from build123d import *

# Parameters (mm, degrees)
SKETCH_1_R          = 102
EXTRUDE_1_DEPTH     = 12
SKETCH_2_R          = 69
EXTRUDE_2_DEPTH     = 3
CUT_EXTRUDE_START   = -4
SKETCH_3_R          = 82
SKETCH_3_R_2        = 69
CUT_EXTRUDE_2_DEPTH = 4
SKETCH_4_R          = 63.75
EXTRUDE_3_DEPTH     = 1
CHAMFER_1_SIZE      = 0.5
SKETCH_5_R          = 5
CUT_EXTRUDE_3_DEPTH = 41
SKETCH_6_R          = 55
CUT_EXTRUDE_4_DEPTH = 51
SKETCH_7_R          = 4
CUT_EXTRUDE_5_DEPTH = 8


with BuildPart() as part:
    # 草图1 → 拉伸1 (new body)
    with BuildSketch(Plane.XY):
        Circle(SKETCH_1_R)
    extrude(amount=EXTRUDE_1_DEPTH)

    # 草图2 → 拉伸2 (add)
    with BuildSketch(Plane.XY.offset(12)):
        Circle(SKETCH_2_R)
    extrude(amount=EXTRUDE_2_DEPTH)

    # 草图3 → 切除-拉伸2 (cut)
    with BuildSketch(Plane.XY.offset(12).offset(CUT_EXTRUDE_START)):
        Circle(SKETCH_3_R)
        Circle(SKETCH_3_R_2, mode=Mode.SUBTRACT)
    extrude(amount=CUT_EXTRUDE_2_DEPTH, mode=Mode.SUBTRACT)

    # 草图4 → 拉伸3 (add)
    with BuildSketch(Plane.XY.offset(15)):
        Circle(SKETCH_4_R)
    extrude(amount=EXTRUDE_3_DEPTH)

    # 倒角1
    chamfer_1_edges = [part.edges().sort_by_distance(p)[0] for p in [
        (-82, 0, 12),
        (-102, 0, 0),
        (-102, 0, 12),
        (-69, 0, 15),
    ]]
    chamfer(chamfer_1_edges, length=CHAMFER_1_SIZE)

    # 草图5 → 切除-拉伸3 (cut)
    with BuildSketch(Plane(origin=(0, 0, 0), x_dir=(-1, 0, 0), z_dir=(0, 0, -1))):
        with Locations((0, 90)):
            Circle(SKETCH_5_R)
        with Locations((77.942286341, 45)):
            Circle(SKETCH_5_R)
        with Locations((77.942286341, -45)):
            Circle(SKETCH_5_R)
        with Locations((0, -90)):
            Circle(SKETCH_5_R)
        with Locations((-77.942286341, -45)):
            Circle(SKETCH_5_R)
        with Locations((-77.942286341, 45)):
            Circle(SKETCH_5_R)
    extrude(amount=-CUT_EXTRUDE_3_DEPTH, mode=Mode.SUBTRACT)

    # 草图6 → 切除-拉伸4 (cut)
    with BuildSketch(Plane(origin=(0, 0, 0), x_dir=(-1, 0, 0), z_dir=(0, 0, -1))):
        Circle(SKETCH_6_R)
    extrude(amount=-CUT_EXTRUDE_4_DEPTH, mode=Mode.SUBTRACT)

    # 草图7 → 切除-拉伸5 (cut)
    with BuildSketch(Plane(origin=(0, 0, 0), x_dir=(-1, 0, 0), z_dir=(0, 0, -1))):
        with Locations((51.265241636, 51.265241636)):
            Circle(SKETCH_7_R)
        with Locations((51.265241636, -51.265241636)):
            Circle(SKETCH_7_R)
        with Locations((-51.265241636, -51.265241636)):
            Circle(SKETCH_7_R)
        with Locations((-51.265241636, 51.265241636)):
            Circle(SKETCH_7_R)
    extrude(amount=-CUT_EXTRUDE_5_DEPTH, mode=Mode.SUBTRACT)


solid = part.part
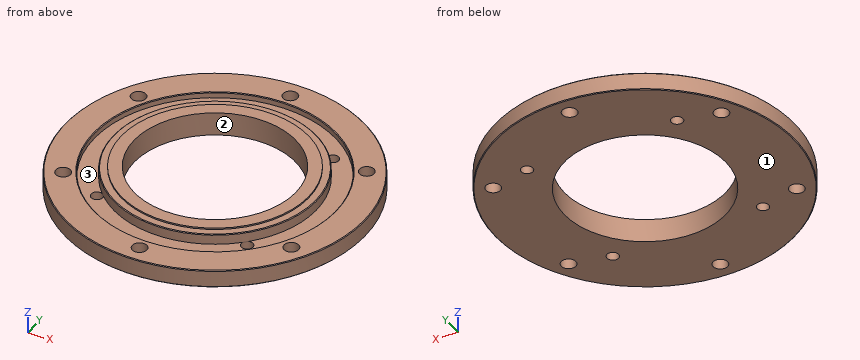
For this review, take the finished solid that the model builds, in its own axes (mm). Face numbers are marked on the shaded views. Round coordinates to 2 decimals unless told otherwise and drop trailing zeros. Loops run counter-clockwise (first coordinate to the right, second up) from the corner with the lowest first, then second, coordinate; pieces in that order, holes last. Notation, with made-up numbers: (-4.5, 66) - (8.5, 66) arc R25 cw to (8.5, 84) - close; hole circle Ø1 at (67, -26). An arc over 180 degrees is marked (long way). Use one line per item in the form item = value.
Item 1: Consider section B-B on z = 4. State how many separate pieces and enclosed holes the cut face has, then the cut area to 3 significant figures.
Answers:
separate_pieces = 1
enclosed_holes = 11
area = 22,500 mm^2
Item 2: Clearance check with flat-ended pins moving along their axes: P1, Ø11.5, axis at x = -77.94, y = -45, coming from the +Z side; P2, Ø3, axis at y = -42, z = 7.5, coming from the +X side; P3, Ø6, axis at y = -77, z = 10.5, coming from the -X side. State where each tip first meets the part, or that it passes through.
Answers:
P1 = 12
P2 = 93.61
P3 = -70.2
Item 3: Mouldability with a two-part tool opening along Y and no side actions: class the marked faces 1, 2 and 3 as +Y half, -Y half, draft (parallel to the pull), parting line (faces both ways), or undercut.
Answers:
face_1 = draft
face_2 = undercut
face_3 = undercut
Item 4: For line 1 (Y direction, x = 0, z = 7); line 2 (Y direction, x = 0, z = 9.7); line 3 (X direction, y = -27, z = 11), list the stretches that pass through material, from the lowest coordinate up.
Answers:
line_1 = -102 to -95, -85 to -55, 55 to 85, 95 to 102
line_2 = -102 to -95, -85 to -82, -69 to -55, 55 to 69, 82 to 85, 95 to 102
line_3 = -98.36 to -77.43, -63.5 to -47.92, 47.92 to 63.5, 77.43 to 98.36
Item 5: Consider section A-A on y = 0. Write out the cut boundary in (x, z).
Answers:
outline = (-102, 0.5) - (-101.5, 0) - (-55, 0) - (-55, 16) - (-63.75, 16) - (-63.75, 15) - (-68.5, 15) - (-69, 14.5) - (-69, 8) - (-82, 8) - (-82, 11.5) - (-82.5, 12) - (-101.5, 12) - (-102, 11.5) - close; (55, 0) - (101.5, 0) - (102, 0.5) - (102, 11.5) - (101.5, 12) - (82.5, 12) - (82, 11.5) - (82, 8) - (69, 8) - (69, 14.5) - (68.5, 15) - (63.75, 15) - (63.75, 16) - (55, 16) - close
